from build123d import *

# Parameters (mm, degrees)
ESQUISSE1_R             = 1
ESQUISSE1_R_2           = 1.2
ESQUISSE1_R_3           = 1.5
BOSS_EXTRU_1_DEPTH      = 5
ENL_V_MAT_EXTRU_1_DEPTH = 108.186752913
CONG_1_R                = 1


with BuildPart() as part:
    # Esquisse1 → Boss.-Extru.1 (new body)
    with BuildSketch(Plane.XY):
        Polygon((-67, 5), (-67, 0), (-90, 0), (-90, -4), (-62, -4), (-62, -52), (-70.4817, -52), (-70.4817, -58), (-62, -58), (90, -58), (90, 0), (75, 0), (75, 5), (70, 5), (70, 0), (66.5, 0), (66.5, -3), (67.6, -3), (67.6, -5.3), (66.5, -5.3), (66.5, -10), (63.5, -10), (63.5, -5.3), (62.4, -5.3), (62.4, -3), (63.5, -3), (63.5, 0), (60, 0), (60, 5), (55, 5), (55, 0), (-47, 0), (-47, 5), (-52, 5), (-52, 0), (-55.5, 0), (-55.5, -3), (-54.4, -3), (-54.4, -5.3), (-55.5, -5.3), (-55.5, -10), (-58.5, -10), (-58.5, -5.3), (-59.6, -5.3), (-59.6, -3), (-58.5, -3), (-58.5, 0), (-62, 0), (-62, 5), align=None)
        with Locations((-67.4817, -55)):
            Circle(ESQUISSE1_R, mode=Mode.SUBTRACT)
        with Locations((42.5183, -55)):
            Circle(ESQUISSE1_R, mode=Mode.SUBTRACT)
        with Locations((-51.30915, -6)):
            Circle(ESQUISSE1_R_2, mode=Mode.SUBTRACT)
        with Locations((-39.3683, -5)):
            Circle(ESQUISSE1_R_3, mode=Mode.SUBTRACT)
        with Locations((29.6317, -5)):
            Circle(ESQUISSE1_R_3, mode=Mode.SUBTRACT)
        with Locations((78.19085, -6)):
            Circle(ESQUISSE1_R_2, mode=Mode.SUBTRACT)
    extrude(amount=BOSS_EXTRU_1_DEPTH)

    # Esquisse2 → Enlèv. mat.-Extru.1 (cut, through all)
    with BuildSketch(Plane(origin=(0, 0, 0), x_dir=(-1, 0, 0), z_dir=(0, 0, -1))):
        Polygon((-90, -16.277013327), (-87.46, -17.201497722), (-87.46, -22.201497722), (-85.46, -22.201497722), (-85.46, -16.652424864), (-90, -15), align=None)
        with BuildLine():
            Line((-76.19085, -6), (-76.19085, -11))
            ThreePointArc((-76.19085, -11), (-78.19085, -13), (-80.19085, -11))
            Line((-80.19085, -11), (-80.19085, -6))
            ThreePointArc((-80.19085, -6), (-78.19085, -4), (-76.19085, -6))
        make_face()
        with BuildLine():
            Line((-76.19085, -48), (-76.19085, -53))
            ThreePointArc((-76.19085, -53), (-78.19085, -55), (-80.19085, -53))
            Line((-80.19085, -53), (-80.19085, -48))
            ThreePointArc((-80.19085, -48), (-78.19085, -46), (-76.19085, -48))
        make_face()
    extrude(amount=-ENL_V_MAT_EXTRU_1_DEPTH, mode=Mode.SUBTRACT)

    # Congé1
    cong_1_edges = [part.edges().sort_by_distance(p)[0] for p in [
        (85.46, -16.652424864, 2.5),
        (90, -15, 2.5),
        (90, -16.277013327, 2.5),
        (87.46, -17.201497722, 2.5),
        (87.46, -22.201497722, 2.5),
        (85.46, -22.201497722, 2.5),
        (90, -58, 2.5),
        (90, 0, 2.5),
        (-90, 0, 2.5),
        (-90, -4, 2.5),
        (-62, -4, 2.5),
        (-62, -52, 2.5),
        (-70.4817, -58, 2.5),
        (-70.4817, -52, 2.5),
    ]]
    fillet(cong_1_edges, radius=CONG_1_R - 0.0001)  # a hair under: the kernel refuses the full size


solid = part.part
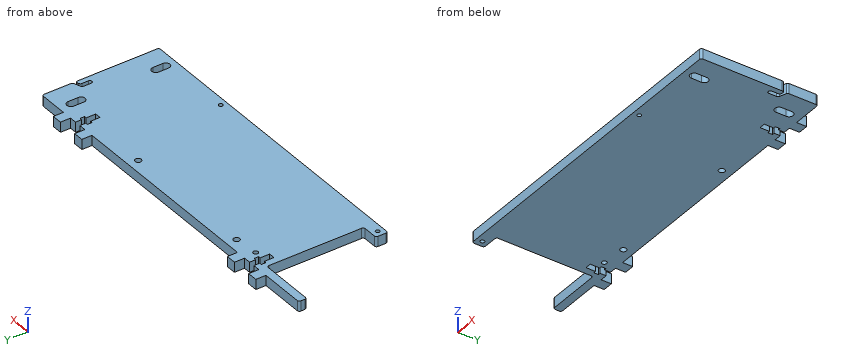
Read the model definition and answer for the solid it produces. Units are mm, in the model's axes. Round coordinates to 2 decimals unless told otherwise and drop trailing zeros. Order: outer loops, then holes, each group sorted by start corner. A loop starts at its lowest first (then second) coordinate and runs counter-clockwise, first axis right, second up.
1) The part is cut by section C-C on z = 1.8. Give the number of separate pieces and of enclosed holes in the cut face, plus the area to 3 significant figures.
2) The part is cut by section B-B on y = -34. Write down the section's boundary in (x, z).
3) Straight lines are drawn through the part: L1, parallel to X at y = -1, z = 0.35; L2, parallel to Y at x = 34, z = 3.75; L3, parallel to X at y = -23, z = 2.45. For each, find the intervals that lie inside material, in ascending order.
4) The part is cut by section A-A on x = 1. Write down the section's boundary in (y, z).
5) Flat-ended cylindrical pins translate along their axes: pin 1 (1.5 mm diameter, centred on y = -46, z = 2, fed in from -X); pin 2 (1 mm diameter, centred on x = -54.5, z = 2.5, fed in from +Y); pin 3 (1.5 mm diameter, centred on y = 3.5, z = 3.5, fed in from +X). Find the tip coordinate at first contact, or state that the pin passes through.
Resolved:
1. separate pieces: 1
1. enclosed holes: 7
1. area: 8,900 mm2
2. outline: (-62, 0) - (90, 0) - (90, 5) - (-62, 5) - close
3. L1: x = -90 to -58.5, -55.5 to 63.5, 66.5 to 90
3. L2: y = -58 to 0
3. L3: x = -62 to 90
4. outline: (-58, 0) - (0, 0) - (0, 5) - (-58, 5) - close
5. pin 1: stops at x = -62
5. pin 2: stops at y = 0
5. pin 3: stops at x = 75
